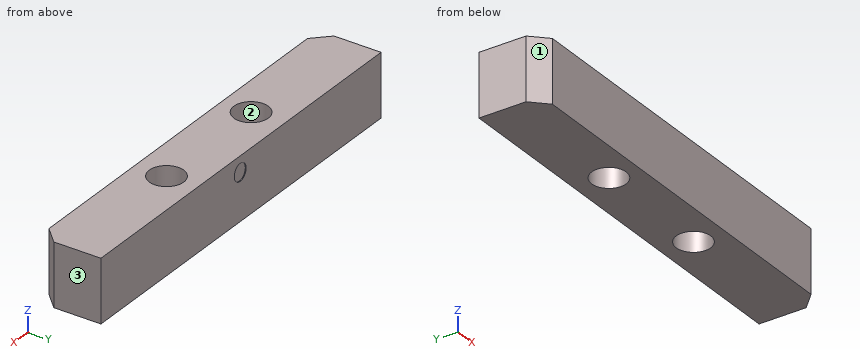
from build123d import *

# Parameters (mm, degrees)
F0_R     = 5.5
F2_DEPTH = 20
F4_D     = 5.5
F4_DEPTH = 12
F4_TIP   = 1.6523667023


# Not quite as in the source:
# - the program builds the solid bodies; features that only make, move or delete a surface that nothing else refers to are left out


with BuildPart() as f2:
    # F0 (on Top) → F2 (new body)
    with BuildSketch(Plane.XY):
        Polygon((64.6278701635, 0.2722779787), (-65.3721298365, 0.2722779787), (-65.3721298365, -14.7277220213), (-60.3721298365, -19.7277220213), (59.6278701635, -19.7277220213), (64.6278701635, -14.7314790532), align=None)
        with Locations((-20.3721298365, -10.2438455071)):
            Circle(F0_R, mode=Mode.SUBTRACT)
        with Locations((19.6245402317, -9.7277220213)):
            Circle(F0_R, mode=Mode.SUBTRACT)
    extrude(amount=F2_DEPTH)

    # F4 (one way)
    with BuildSketch(Plane.XZ):
        with Locations((0, 15)):
            Circle(F4_D / 2)
    extrude(amount=-F4_DEPTH, mode=Mode.SUBTRACT)
    with Locations(Plane.XZ):
        with Locations((0, 15)):
            with Locations((0, 0, -(F4_DEPTH + F4_TIP / 2))):  # 118° drill point
                Cone(0, F4_D / 2, F4_TIP, mode=Mode.SUBTRACT)


solid = f2.part
Here's how the part is built. I have some questions about the finished solid (model axes, mm). Face numbers are marked on the shaded views. Round coordinates to 2 decimals unless told otherwise and drop trailing zeros. Loops run counter-clockwise (first coordinate to the right, second up) from the corner with the lowest first, then second, coordinate; pieces in that order, holes last. Notation, with made-up numbers: M 84,-34.75 L 96,-34.75 A25 ccw 96,-9.75 Z; hole C 48.5,65 d11. An arc over 180 degrees is marked long. Write each question's results on one line, items separated by ' | '. Start each with the question number.
(1) If I drill on probe 1 along X at (y, z) = (-6.75, 17.75); probe 2 along X at (y, z) = (-6, 5); probe 3 along Y at (x, z) = (-23.5, 14.5), over which ranges is the centre line in solid material (lowest first)? Write a range as from..to.
(2) I want a section at C-C (x = -16.5). Please give me the cut outline in (y, z), then the cut area to 3 significant figures.
(3) I want a section at A-A (y = -7.25). Please give me the cut outline in (x, z), then the cut area to 3 significant figures.
(4) Thinking about a two-plate mould opening in Y: for the marked faces 1, 2 and 3, which applies, pulls with the +Y half, pulls with the -Y half, needs draft (parallel to the pull), parting line crosses it, or undercut?
(5) Will these pins go through, and if not, where does the flat tip stop? P1, Ø10, axis at x = 19.62, y = -9.73, coming from the +Z side; P2, Ø1.5, axis at x = 1.5, z = 14, coming from the +Y side.
(6) I want a section at B-B (z = 15). Please give me the cut outline in (x, y).
(7) I want a section at D-D (y = -12). Please give me the cut outline in (x, z).
Solved:
1) probe 1: x = -65.37..-24.62, -16.12..15, 24.25..64.63 | probe 2: x = -65.37..-23.87, -16.87..15.58, 23.67..64.63 | probe 3: y = -19.73..-14.77, -5.72..0.27
2) outline: M -19.73,0 L -14.15,0 L -14.15,20 L -19.73,20 Z; M -6.34,0 L 0.27,0 L 0.27,20 L -6.34,20 Z | area: 244 mm²
3) outline: M -65.37,0 L -24.99,0 L -24.99,20 L -65.37,20 Z; M -15.76,0 L 14.71,0 L 14.71,20 L -15.76,20 Z; M 24.53,0 L 64.63,0 L 64.63,20 L 24.53,20 Z | area: 2,220 mm²
4) face 1: pulls with the -Y half | face 2: undercut | face 3: needs draft
5) P1: passes through | P2: stops at y = 0
6) outline: M -65.37,-14.73 L -60.37,-19.73 L 59.63,-19.73 L 64.63,-14.73 L 64.63,0.27 L 2.75,0.27 L 2.75,0 L -2.75,0 L -2.75,0.27 L -65.37,0.27 Z; hole C -20.37,-10.24 d11; hole C 19.62,-9.73 d11
7) outline: M -65.37,0 L -25.58,0 L -25.58,20 L -65.37,20 Z; M -15.16,0 L 14.62,0 L 14.62,20 L -15.16,20 Z; M 24.63,0 L 64.63,0 L 64.63,20 L 24.63,20 Z
